Geometry: final body of the model. Coordinates: model frame, mm. A direction names the side the tool comes from. Round coordinates to 2 decimals unless told otherwise and drop trailing zeros. Write each loop counter-clockwise with the first axis right and the second up, starting at its lowest first coordinate (ties: lowest second). Pieces come first, ordered by that corner, then holes. Notation, with made-up numbers: M 24,50.5 L 29,50.5 A24 cw 29,64.5 Z; hole C 1,-40 d9. An arc over 180 degrees is marked long. Put each result on its own line as item: value. Start each with the question number.
```python
from build123d import *

# Parameters (mm, degrees)
F0_W     = 6.288823
F0_H     = 22.754102
F0_R     = 4.68301
F1_DEPTH = 10
F2_DEPTH = 13


with BuildPart() as f1:
    # F0 (on Top) → F1 (new body)
    with BuildSketch(Plane.XY):
        with BuildLine():
            Line((20.521231, 4.569745), (20.521231, 31.395026))
            ThreePointArc((20.521231, 31.395026), (13.021231, 50.816255), (5.521231, 31.395026))
            Line((5.521231, 31.395026), (5.521231, 4.569745))
            Line((5.521231, 4.569745), (20.521231, 4.569745))
        make_face()
        with Locations((13.274627, 19.26272)):
            Rectangle(F0_W, F0_H, mode=Mode.SUBTRACT)
        with Locations((13.021231, 39.657483)):
            Circle(F0_R, mode=Mode.SUBTRACT)
    extrude(amount=F1_DEPTH)

    # F0 (on Top) → F2 (join)
    with BuildSketch(Plane.XY):
        with Locations((13.274627, 19.26272)):
            Rectangle(F0_W, F0_H)
    extrude(amount=F2_DEPTH)


solid = f1.part
```
1) Section B-B, the plane z = 1. Output: boundary loops of the cut face in (x, y), and give its area (3 significant figures).
2) Section D-D, the plane y = 38. Output: boundary loops of the cut face in (x, z), and give its area (3 significant figures).
3) Ray query, probe 1 along X at (y, z) = (14.5, 12); probe 2 along Z at (x, y) = (16, 45); probe 3 along Y at (x, z) = (10.5, 5.5). Return the intervals inside material, ascending.
4) Section A-A, the plane x = 12. Output: boundary loops of the cut face in (y, z), and give its area (3 significant figures).
5) Draft query along Y for faces 1 (the face through (12.4, 44.3, 4.9)), 2 (the face through (13, 30.64, 11)), 3 (the face through (13, 7.886, 11)), 4 (the face through (10.13, 19, 11)). Return one class per face: +Y half, -Y half, draft (parallel to the pull), parting line (faces both ways), or undercut.
6) Access query for faces 5 (the face through (20.521, 18, 5)), 6 (the face through (5.521, 18, 5)), 7 (the face through (16.419, 19, 11)). Directions: +Z, -Z, +X, -X, +Y, -Y. A direction counts if a zero-diameter tool reaches every point of the face in a straight line with its end or side. Return the directions, or none.
7) First-contact query: pin 1 (6 mm diameter, centred on y = 11.5, z = 5, fed in from +X); pin 2 (1.5 mm diameter, centred on x = 13, z = 11, fed in from +Y); pin 3 (2.5 mm diameter, centred on x = 14, z = 12, fed in from -Y). Flat tips, straight axial feed; report the tip coordinate or a pass-through.
8) Section C-C, the plane y = 9. Output: boundary loops of the cut face in (x, z), and give its area (3 significant figures).
Solved:
1. outline: M 5.52,4.57 L 20.52,4.57 L 20.52,31.4 A11.16 ccw long 5.52,31.4 Z; hole C 13.02,39.66 d9.37
1. area: 695 mm2
2. outline: M 1.99,0 L 8.64,0 L 8.64,10 L 1.99,10 Z; M 17.4,0 L 24.06,0 L 24.06,10 L 17.4,10 Z
2. area: 133 mm2
3. probe 1: x = 10.13 to 16.42
3. probe 2: z = 0 to 10
3. probe 3: y = 4.57 to 35.71, 43.6 to 50.53
4. outline: M 4.57,0 L 35.09,0 L 35.09,10 L 30.64,10 L 30.64,13 L 7.89,13 L 7.89,10 L 4.57,10 Z; M 44.23,0 L 50.77,0 L 50.77,10 L 44.23,10 Z
4. area: 439 mm2
5. face 1: undercut
5. face 2: +Y half
5. face 3: -Y half
5. face 4: draft
6. face 5: +Z, -Z, +X, -Y
6. face 6: +Z, -Z, -X, -Y
6. face 7: +Z, +X, +Y, -Y
7. pin 1: stops at x = 20.52
7. pin 2: stops at y = 30.64
7. pin 3: stops at y = 7.89
8. outline: M 5.52,0 L 20.52,0 L 20.52,10 L 16.42,10 L 16.42,13 L 10.13,13 L 10.13,10 L 5.52,10 Z
8. area: 169 mm2
